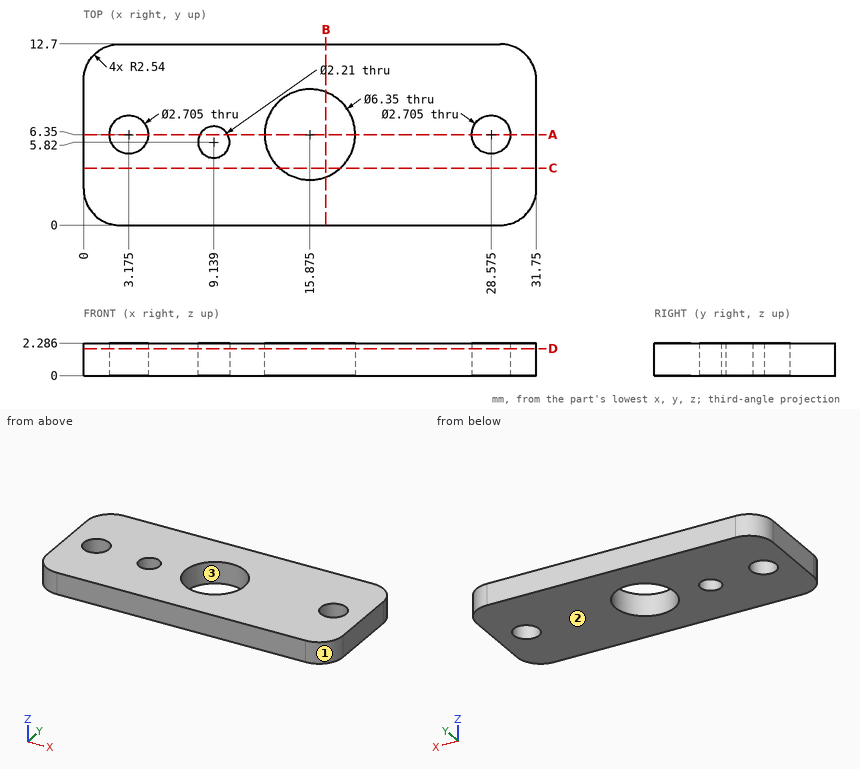
Input: dimensioned drawing with shaded views. Units: mm. Origin: part minimum x, y, z. Coordinates: 2 decimals unless noted, no trailing zeros. Loops run counter-clockwise (first coordinate to the right, second up) from the corner with the lowest first, then second, coordinate; pieces in that order, holes last. Notation, with made-up numbers: M 16,15 L 28,15 A19 cw 28,49 Z; hole C 50.5,-37 d5. An arc over 180 degrees is marked long. Put each result on its own line as item: value.
(1) Cut plane D-D on z = 1.9. State how many separate pieces and enclosed holes the cut face has, then the cut area to 3 significant figures.
Answer sheet:
separate pieces: 1
enclosed holes: 4
area: 351 mm^2
(2) Draft query along X for the marked faces 1, 2 and 3. Return one class per face: pulls with the +X half, pulls with the -X half, needs draft (parallel to the pull), parting line crosses it, or undercut.
Answer sheet:
face 1: pulls with the +X half
face 2: needs draft
face 3: undercut
(3) Material intervals for probe 1 along X at (y, z) = (6.35, 1.15); probe 2 along Y at (x, z) = (2, 0.7) (1 decimal); probe 3 along Y at (x, z) = (29, 0.2) (1 decimal), sorted ascending.
Answer sheet:
probe 1: x = 0 to 1.82, 4.53 to 8.17, 10.11 to 12.7, 19.05 to 27.22, 29.93 to 31.75
probe 2: y = 0.1 to 5.7, 7 to 12.6
probe 3: y = 0 to 5.1, 7.6 to 12.7
(4) Cut plane C-C on y = 4. Return the cut outline in (x, z).
Answer sheet:
outline: M 0,0 L 13.74,0 L 13.74,2.29 L 0,2.29 Z; M 18.01,0 L 31.75,0 L 31.75,2.29 L 18.01,2.29 Z
(5) Cut plane A-A on y = 6.35. Return the cut outline in (x, z).
Answer sheet:
outline: M 0,0 L 1.82,0 L 1.82,2.29 L 0,2.29 Z; M 4.53,0 L 8.17,0 L 8.17,2.29 L 4.53,2.29 Z; M 10.11,0 L 12.7,0 L 12.7,2.29 L 10.11,2.29 Z; M 19.05,0 L 27.22,0 L 27.22,2.29 L 19.05,2.29 Z; M 29.93,0 L 31.75,0 L 31.75,2.29 L 29.93,2.29 Z
(6) Cut plane B-B on x = 17. Return the cut outline in (y, z).
Answer sheet:
outline: M 0,0 L 3.38,0 L 3.38,2.29 L 0,2.29 Z; M 9.32,0 L 12.7,0 L 12.7,2.29 L 9.32,2.29 Z
